Job drawing, mm, ordinate dimensions from the low corner. One solid piece. Round coordinates to 2 decimals unless told otherwise and drop trailing zeros. Loops run counter-clockwise (first coordinate to the right, second up) from the corner with the lowest first, then second, coordinate; pieces in that order, holes last. Notation, with made-up numbers: M 78.25,-5 L 98.25,-5 A21 ccw 98.25,5 Z; hole C 4,-28 d7. An arc over 180 degrees is marked long. Put each result on its own line as item: value. Start each with the question number.
1) Slice it at B-B on x = 54. Give the cut face in (y, z) (1 decimal), then the cut area to 3 significant figures.
2) Pull direction Y, two halves, no side cores. Call the marked faces 1, 2 and 3: +Y half, -Y half, draft (parallel to the pull), parting line (faces both ways), or undercut.
3) Drop flat-ended pins along their axis: pin 1 Ø3 at (y, z) = (8.5, 5.5) entering from -X; pin 2 Ø0.9 at (y, z) = (23, 8.5) entering from -X; pin 3 Ø4.5 at (x, z) = (33.5, 1.5) entering from +Y; pin 4 Ø1.5 at (y, z) = (22.5, 7.5) entering from +X. Give the stop position or say it passes through.
4) Slice it at A-A on z = 6. Give the cut face in (x, y) (1 decimal).
5) Probe line 1 along Y through (x, z) = (56, 5) (1 decimal); line 2 along Z through (x, y) = (57.5, 20); line 3 along Y through (x, z) = (3, 1.25). List the from-to ranges inside material, lowest first.
6) Slice it at C-C on z = 3. Give the cut face in (x, y) (1 decimal).
7) Slice it at D-D on y = 12.5. Give the cut face in (x, z).
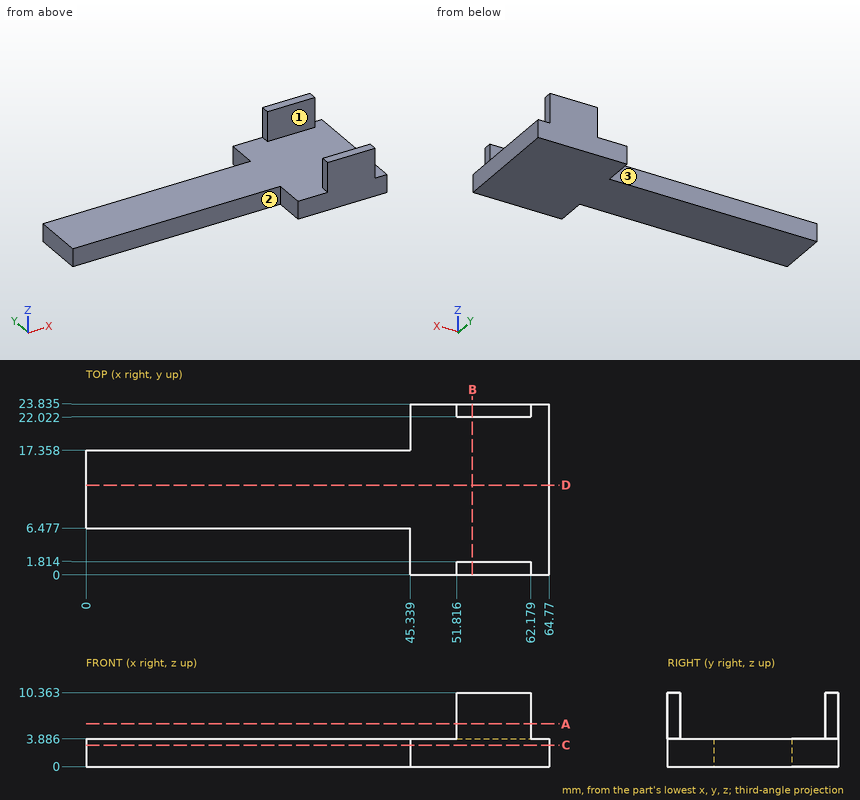
Recorded:
1. outline: M 0,0 L 23.8,0 L 23.8,10.4 L 22,10.4 L 22,3.9 L 1.8,3.9 L 1.8,10.4 L 0,10.4 Z
1. area: 116 mm2
2. face 1: undercut
2. face 2: -Y half
2. face 3: +Y half
3. pin 1: passes through
3. pin 2: stops at x = 51.82
3. pin 3: stops at y = 17.36
3. pin 4: stops at x = 62.18
4. outline: M 51.8,0 L 62.2,0 L 62.2,1.8 L 51.8,1.8 Z; M 51.8,22 L 62.2,22 L 62.2,23.8 L 51.8,23.8 Z
5. line 1: y = 0 to 1.8, 22 to 23.8
5. line 2: z = 0 to 3.89
5. line 3: y = 6.48 to 17.36
6. outline: M 0,6.5 L 45.3,6.5 L 45.3,0 L 64.8,0 L 64.8,23.8 L 45.3,23.8 L 45.3,17.4 L 0,17.4 Z
7. outline: M 0,0 L 64.77,0 L 64.77,3.89 L 0,3.89 Z
